Could you check a few things on this drawing? It's one solid part, dimensions in mm from its lowest x, y, z. A direction names the side the tool comes from. Give positions to 0.01 mm unless a question says otherwise; leave off trailing zeros. Order: outer loops, then holes, each group sorted by start corner. A loop starts at its lowest first (then second) coordinate and runs counter-clockwise, first axis right, second up. Notation, with made-up numbers: (-0.5, -11.5) - (26.5, -11.5) arc R24 ccw to (26.5, 8.5) - close; hole circle Ø5 at (19.25, -2). An arc over 180 degrees is marked (long way). Answer as CSV lines item,"result".
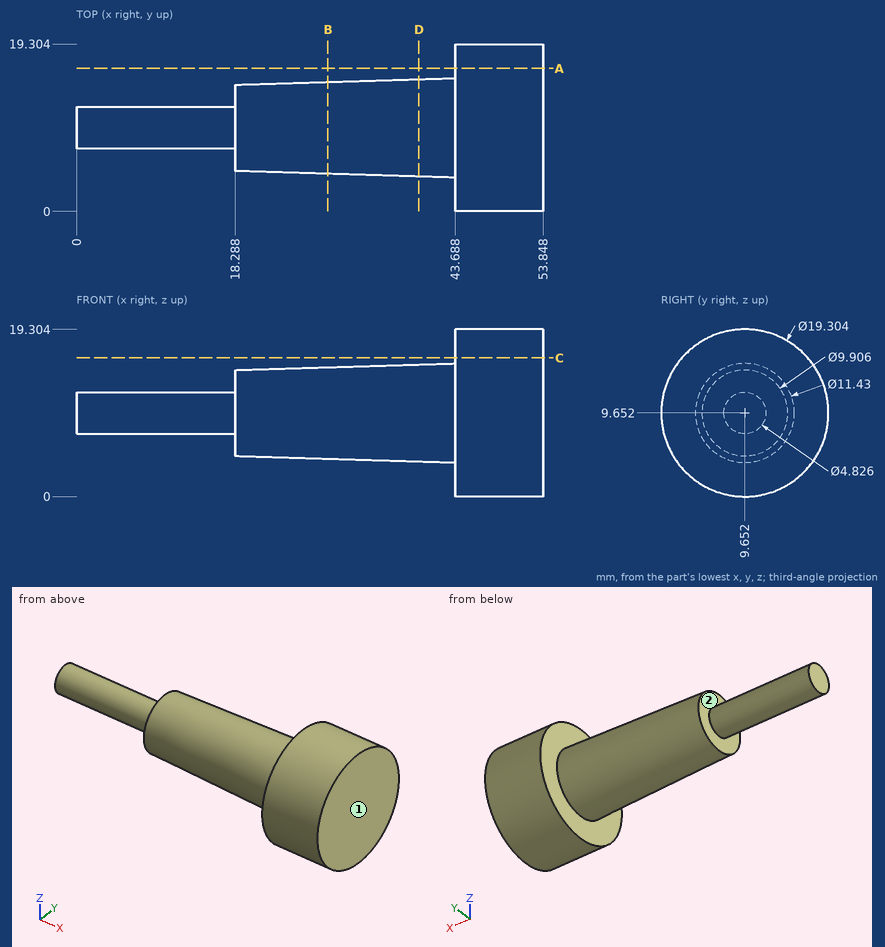
1) I want a section at A-A on y = 16.5. Write out the boundary of the cut face in (x, z), plus the area to 3 significant figures.
Answer block:
outline,"(43.69, 2.85) - (53.85, 2.85) - (53.85, 16.45) - (43.69, 16.45) - close"
area,"138 mm2"
2) I want a section at B-B on x = 29. Write out the boundary of the cut face in (y, z), plus the area to 3 significant figures.
Answer block:
outline,"circle Ø10.55 at (9.65, 9.65)"
area,"87.4 mm2"
3) Which directions (+Z, -Z, +X, -X, +Y, -Y) give clear straight access to the entire face, cutting with the end or side of a thin tool? Please do the marked faces 1 and 2.
Answer block:
face 1,"+Z, -Z, +X, +Y, -Y"
face 2,"-X"
4) I want a section at C-C on z = 16. Write out the boundary of the cut face in (x, y), plus the area to 3 significant figures.
Answer block:
outline,"(43.69, 2.38) - (53.85, 2.38) - (53.85, 16.92) - (43.69, 16.92) - close"
area,"148 mm2"
5) I'm going to push flat-ended pins straight in: P1, Ø5, axis at x = 6, z = 17, coming from the +Y side; P2, Ø6, axis at y = 3, z = 3, coming from the -X side. Where does each tip first touch, or does it pass through?
Answer block:
P1,"through"
P2,"x = 43.69"
6) I want a section at D-D on x = 39.5. Write out the boundary of the cut face in (y, z), plus the area to 3 significant figures.
Answer block:
outline,"circle Ø11.18 at (9.65, 9.65)"
area,"98.1 mm2"
7) I need wall thicknesses on line 1 along X through (y, z) = (1.75, 5); line 2 along X through (y, z) = (10.75, 6.75); line 3 along Z through (x, y) = (19, 10). Which ranges of each line are inside material? Lowest first, please. Write a range as [from, to].
Answer block:
line 1,"[43.69, 53.85]"
line 2,"[18.29, 53.85]"
line 3,"[4.69, 14.61]"
